For this review, take the finished solid that the model builds, in its own axes (mm). Face numbers are marked on the shaded views. A direction names the side the tool comes from. Give positions to 0.01 mm unless a question says otherwise; leave off trailing zeros. Order: outer loops, then holes, each group sorted by start corner. A loop starts at its lowest first (then second) coordinate and runs counter-clockwise, first axis right, second up. Notation, with made-up numbers: (65, -18) - (94, -18) arc R27 ccw to (94, 13) - close; hole circle Ø7 at (38, -27). An arc over 180 degrees is marked (long way). One line per item, written item: value.
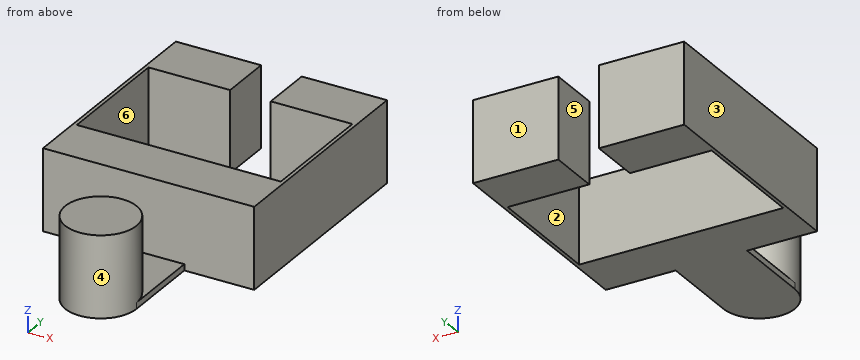
```python
from build123d import *

# Parameters (mm, degrees)
SKETCH1_R           = 11.162804955
BOSS_EXTRUDE1_DEPTH = 25.4
BOSS_EXTRUDE2_START = -1.926431551
BOSS_EXTRUDE2_DEPTH = 1.926431551
SKETCH4_W           = 66.04
SKETCH4_H           = 25.4
BOSS_EXTRUDE3_DEPTH = 16.064370514
SKETCH5_W           = 1.129641984
SKETCH5_H           = 25.4
BOSS_EXTRUDE4_DEPTH = 38.1
SKETCH6_W           = 26.67
SKETCH6_H           = 25.4
BOSS_EXTRUDE5_DEPTH = 16.461081374


with BuildPart() as part:
    # Sketch1 → Boss-Extrude1 (new body)
    with BuildSketch(Plane.XY):
        Circle(SKETCH1_R)
    extrude(amount=-BOSS_EXTRUDE1_DEPTH)

    # Sketch2 → Boss-Extrude2 (add)
    with BuildSketch(Plane(origin=(0, 0, -25.4), x_dir=(-1, 0, 0), z_dir=(0, 0, -1)).offset(BOSS_EXTRUDE2_START)):
        with BuildLine():
            Line((-11.162804955, 0), (-11.162804955, 25.4))
            Line((-11.162804955, 25.4), (11.162804955, 25.4))
            Line((11.162804955, 25.4), (11.162804955, 0))
            ThreePointArc((11.162804955, 0), (0, 11.162804955), (-11.162804955, 0))
        make_face()
    extrude(amount=BOSS_EXTRUDE2_DEPTH)

    # Sketch4 → Boss-Extrude3 (add)
    with BuildSketch(Plane(origin=(0, 25.4, 0), x_dir=(1, 0, 0), z_dir=(0, 1, 0))):
        with Locations((0, 12.7)):
            Rectangle(SKETCH4_W, SKETCH4_H)
    extrude(amount=BOSS_EXTRUDE3_DEPTH)

    # Sketch5 → Boss-Extrude4 (add)
    with BuildSketch(Plane(origin=(0, 41.464370514, 0), x_dir=(1, 0, 0), z_dir=(0, 1, 0))):
        with Locations((-32.455179008, 12.7)):
            Rectangle(SKETCH5_W, SKETCH5_H)
        with Locations((32.455179008, 12.7)):
            Rectangle(SKETCH5_W, SKETCH5_H)
    extrude(amount=BOSS_EXTRUDE4_DEPTH)

    # Sketch6 → Boss-Extrude5 (add)
    with BuildSketch(Plane(origin=(0, 79.564370514, 0), x_dir=(1, 0, 0), z_dir=(0, 1, 0))):
        with Locations((19.685, 12.7)):
            Rectangle(SKETCH6_W, SKETCH6_H)
        with Locations((-19.685, 12.7)):
            Rectangle(SKETCH6_W, SKETCH6_H)
    extrude(amount=BOSS_EXTRUDE5_DEPTH)


solid = part.part
```
(1) Take a section at A-A (z = -19.25). Write out the cut boundary in (x, y), then the cut area to 3 significant figures.
Answers below:
outline: (-33.02, 25.4) - (33.02, 25.4) - (33.02, 96.03) - (6.35, 96.03) - (6.35, 79.56) - (31.89, 79.56) - (31.89, 41.46) - (-31.89, 41.46) - (-31.89, 79.56) - (-6.35, 79.56) - (-6.35, 96.03) - (-33.02, 96.03) - close; circle Ø22.33 at (0, 0)
area: 2,420 mm^2
(2) For P1, Ø0.6, axis at y = 14.5, z = -25, coming from the +X side; P2, Ø1, axis at y = 16, z = -24, coming from the -X side; P3, Ø8, axis at x = 16, z = -8, coming from the -Y side, all flat-tipped, find the tip position at first contact; note any pin that passes through.
Answers below:
P1: stops at x = 11.16
P2: stops at x = -11.16
P3: stops at y = 25.4
(3) Wall thickness on line 1 (Y direction, x = 25.5, z = -8.25); line 2 (X direction, y = 76, z = -7.5); line 3 (Y direction, x = -6.5, z = -21.5): over which ranges is each line inside the solid? List them lowest first. Write a range as from..to.
Answers below:
line 1: y = 25.4..41.46, 79.56..96.03
line 2: x = -33.02..-31.89, 31.89..33.02
line 3: y = -9.08..9.08, 25.4..41.46, 79.56..96.03
(4) Take a section at D-D (x = 0). Write out the cut boundary in (y, z), then the cut area to 3 significant figures.
Answers below:
outline: (-11.16, -25.4) - (41.46, -25.4) - (41.46, 0) - (25.4, 0) - (25.4, -23.47) - (11.16, -23.47) - (11.16, 0) - (-11.16, 0) - close
area: 1,000 mm^2
(5) Machinability: for the marked faces 4, 5 and 6, which of the approach directions +Z, -Z, +X, -X, +Y, -Y give a long, thin tool a straight path to every point of the face, cutting with its end or side? Answer none if there is none.
Answers below:
face 4: +Z
face 5: +Z, -Z, +Y
face 6: +Z, -Z
(6) Draft analysis for pull direction Y (two halves, no side actions). For the marked faces 1, 2 and 3, state which applies: pulls with the +Y half, pulls with the -Y half, needs draft (parallel to the pull), parting line crosses it, or undercut.
Answers below:
face 1: pulls with the +Y half
face 2: undercut
face 3: needs draft
(7) Take a section at B-B (x = 27.5). Write out the cut boundary in (y, z).
Answers below:
outline: (25.4, -25.4) - (41.46, -25.4) - (41.46, 0) - (25.4, 0) - close; (79.56, -25.4) - (96.03, -25.4) - (96.03, 0) - (79.56, 0) - close
(8) Take a section at C-C (y = 69). Write out the cut boundary in (x, z), then the cut area to 3 significant figures.
Answers below:
outline: (-33.02, -25.4) - (-31.89, -25.4) - (-31.89, 0) - (-33.02, 0) - close; (31.89, -25.4) - (33.02, -25.4) - (33.02, 0) - (31.89, 0) - close
area: 57.4 mm^2
